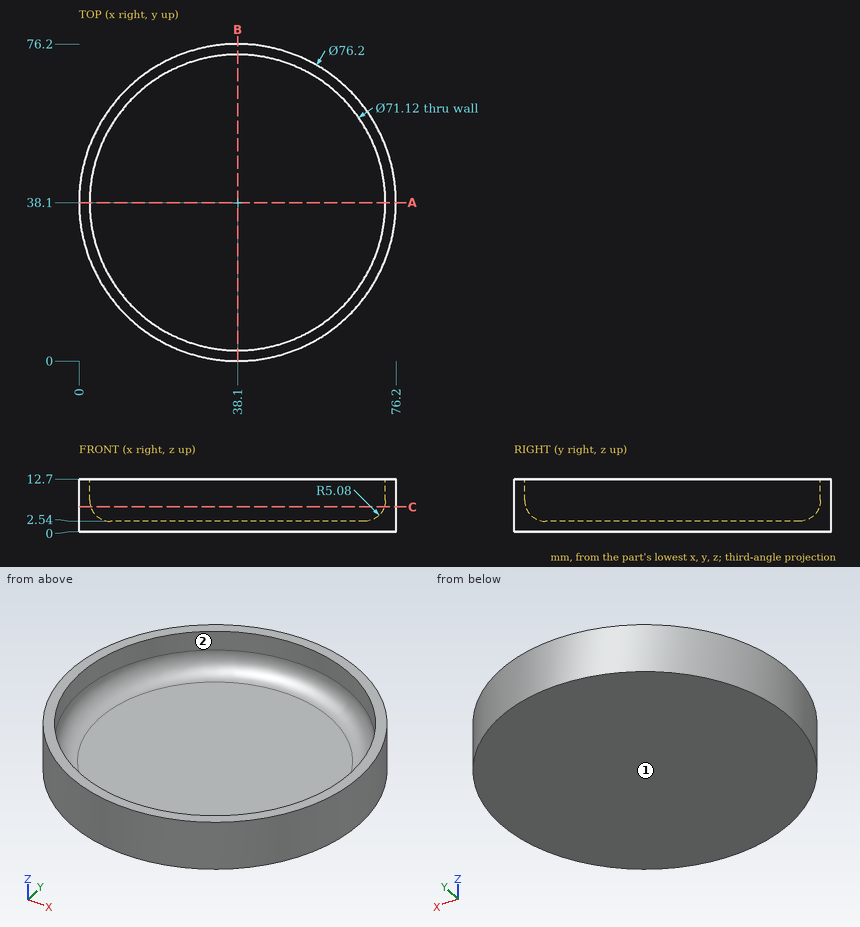
Answer from the drawing. Dimensions are ordinates in mm from the lowest x, y and z of the part. A direction names the side the tool comes from. Round coordinates to 2 decimals unless told otherwise and drop trailing zeros. Order: outer loops, then holes, each group sorted by start corner. A loop starts at its lowest first (then second) coordinate and runs counter-clockwise, first axis right, second up.
1) The part is cut by section C-C on z = 6. Write down the section's boundary in (x, y), plus the area to 3 significant figures.
2) Flat-ended cylindrical pins translate along their axes: pin 1 (5 mm diameter, centred on x = 51.5, z = 5, fed in from +Y); pin 2 (1.5 mm diameter, centred on y = 27.5, z = 9.5, fed in from -X); pin 3 (1 mm diameter, centred on y = 46.5, z = 9.5, fed in from -X). Find the tip coordinate at first contact, or state that the pin passes through.
3) Straight lines are drawn through the part: L1, parallel to Y at x = 38.1, z = 10.6; L2, parallel to Y at x = 64.5, z = 7; L3, parallel to X at y = 59, z = 4.5. For each, find the intervals that lie inside material, in ascending order.
4) The part is cut by section A-A on y = 38.1. Write down the section's boundary in (x, z).
5) For the marked faces 1 and 2, determine the directions among +Z, -Z, +X, -X, +Y, -Y from which every point of the face is accessible in a straight line to the end or side of a thin tool.
Resolved:
1. outline: circle Ø76.2 at (38.1, 38.1); hole circle Ø70.59 at (38.1, 38.1)
1. area: 647 mm2
2. pin 1: stops at y = 74.61
2. pin 2: stops at x = 1.3
2. pin 3: stops at x = 0.83
3. L1: y = 0 to 2.54, 73.66 to 76.2
3. L2: y = 10.63 to 14.33, 61.87 to 65.57
3. L3: x = 6.24 to 10.66, 65.54 to 69.96
4. outline: (0, 0) - (76.2, 0) - (76.2, 12.7) - (73.66, 12.7) - (73.66, 7.62) arc R5.08 cw to (68.58, 2.54) - (7.62, 2.54) arc R5.08 cw to (2.54, 7.62) - (2.54, 12.7) - (0, 12.7) - close
5. face 1: -Z, +X, -X, +Y, -Y
5. face 2: +Z
